Part model, mm, in its own coordinate system. Coordinates: 2 decimals unless noted, no trailing zeros. Write each loop counter-clockwise with the first axis right and the second up, starting at its lowest first coordinate (ties: lowest second). Pieces come first, ordered by that corner, then holes. Notation, with made-up numbers: (-27, 20) - (-5, 20) arc R15 ccw to (-5, 47) - close; hole circle Ø9 at (-34.75, 82.25). An arc over 180 degrees is marked (long way). Use a Markdown table: item, result.
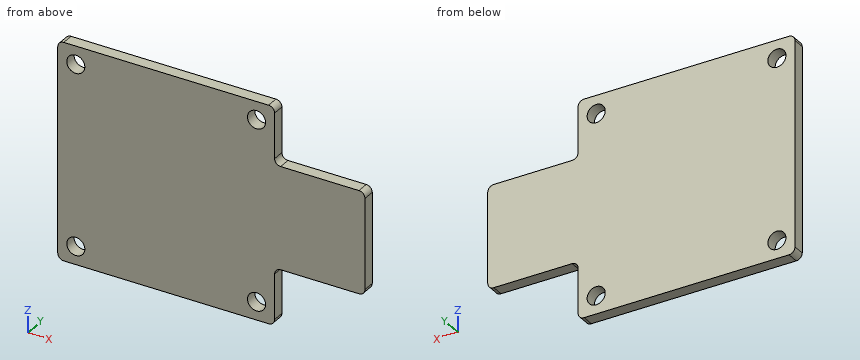
```python
from build123d import *

# Parameters (mm, degrees)
SKETCH1_W           = 36
SKETCH1_H           = 36
SKETCH1_R           = 1.5
SKETCH1_W_2         = 15
SKETCH1_H_2         = 17
BOSS_EXTRUDE1_DEPTH = 2
FILLET1_R           = 1


with BuildPart() as part:
    # Sketch1 → Boss-Extrude1 (new body)
    # profile 1 of 2: a face of its own
    with BuildSketch(Plane(origin=(0, 0, 0), x_dir=(1, 0, 0), z_dir=(0, 1, 0))):
        with Locations((18, 18)):
            Rectangle(SKETCH1_W, SKETCH1_H)
        with Locations(Location((33, 3, 0), (0, 0, 270))):
            Circle(SKETCH1_R, mode=Mode.SUBTRACT)
        with Locations(Location((3, 3, 0), (0, 0, 270))):
            Circle(SKETCH1_R, mode=Mode.SUBTRACT)
        with Locations(Location((33, 33, 0), (0, 0, 270))):
            Circle(SKETCH1_R, mode=Mode.SUBTRACT)
        with Locations(Location((3, 33, 0), (0, 0, 270))):
            Circle(SKETCH1_R, mode=Mode.SUBTRACT)
    # profile 2 of 2: a face of its own
    with BuildSketch(Plane(origin=(0, 0, 0), x_dir=(1, 0, 0), z_dir=(0, 1, 0))):
        with Locations((43.5, 18)):
            Rectangle(SKETCH1_W_2, SKETCH1_H_2)
    extrude(amount=BOSS_EXTRUDE1_DEPTH)

    # Fillet1
    fillet1_edges = [part.edges().sort_by_distance(p)[0] for p in [
        (0, 1, 0),
        (0, 1, -36),
        (36, 1, -36),
        (36, 1, -26.5),
        (51, 1, -26.5),
        (51, 1, -9.5),
        (36, 1, -9.5),
        (36, 1, 0),
    ]]
    fillet(fillet1_edges, radius=FILLET1_R)


solid = part.part
```
Item 1: Band-saw the part on D-D, the plane x = 42. Give the cut face in (y, z).
From the geometry:
| item | result |
|---|---|
| outline | (0, -26.5) - (2, -26.5) - (2, -9.5) - (0, -9.5) - close |
Item 2: Band-saw the part on C-C, the plane x = 33. Give the cut face in (y, z).
From the geometry:
| item | result |
|---|---|
| outline | (0, -36) - (2, -36) - (2, -34.5) - (0, -34.5) - close; (0, -31.5) - (2, -31.5) - (2, -4.5) - (0, -4.5) - close; (0, -1.5) - (2, -1.5) - (2, 0) - (0, 0) - close |
Item 3: Band-saw the part on B-B, the plane z = -33. Give the cut face in (x, y), then the cut area to 3 significant figures.
From the geometry:
| item | result |
|---|---|
| outline | (0, 0) - (1.5, 0) - (1.5, 2) - (0, 2) - close; (4.5, 0) - (31.5, 0) - (31.5, 2) - (4.5, 2) - close; (34.5, 0) - (36, 0) - (36, 2) - (34.5, 2) - close |
| area | 60.0 mm^2 |
Item 4: Drill centre lines: probe 1 along X at (y, z) = (1.2, -33); probe 2 along X at (y, z) = (1.25, -4); probe 3 along X at (y, z) = (0.6, -30.5). Where is each one in solid material? Low to high.
From the geometry:
| item | result |
|---|---|
| probe 1 | 0 to 1.5, 4.5 to 31.5, 34.5 to 36 |
| probe 2 | 0 to 1.88, 4.12 to 31.88, 34.12 to 36 |
| probe 3 | 0 to 36 |
Item 5: Band-saw the part on A-A, the plane y = 1.3. Give the cut face in (x, z), then the cut area to 3 significant figures.
From the geometry:
| item | result |
|---|---|
| outline | (0, -35) arc R1 ccw to (1, -36) - (35, -36) arc R1 ccw to (36, -35) - (36, -27.5) arc R1 cw to (37, -26.5) - (50, -26.5) arc R1 ccw to (51, -25.5) - (51, -10.5) arc R1 ccw to (50, -9.5) - (37, -9.5) arc R1 cw to (36, -8.5) - (36, -1) arc R1 ccw to (35, 0) - (1, 0) arc R1 ccw to (0, -1) - close; hole circle Ø3 at (3, -33); hole circle Ø3 at (3, -3); hole circle Ø3 at (33, -33); hole circle Ø3 at (33, -3) |
| area | 1,520 mm^2 |
Item 6: Drop a flat-ended pin along its axis: P1, Ø1, axis at x = 42, y = 0.5, coming from the +Z side. Give the stop position or say it passes through.
From the geometry:
| item | result |
|---|---|
| P1 | z = -9.5 |
